Model file for the job. Use its own axes, mm. A direction names the side the tool comes from. Round coordinates to 2 decimals unless told otherwise and drop trailing zeros. Loops run counter-clockwise (first coordinate to the right, second up) from the corner with the lowest first, then second, coordinate; pieces in that order, holes last. Notation, with made-up numbers: (-27.75, 58) - (17.25, 58) arc R8 ccw to (17.25, 64) - close; hole circle Ø8 at (-17.75, -15). An arc over 180 degrees is marked (long way). Answer as a JSON object with one key per item and string values.
Autodesk Inventor part; units mm, degrees
ref_plane "YZ Plane" through (0, 0, 0) normal (1, 0, 0) x (0, 1, 0)
ref_plane "XZ Plane" through (0, 0, 0) normal (0, 1, 0) x (-1, 0, 0)
ref_plane "XY Plane" through (0, 0, 0) normal (0, 0, 1) x (1, 0, 0)
sketch "Sketch1" plane through (0, 0, 0) normal (0, 0, 1) x (1, 0, 0)
  line L0 (2.5344, 6.8804) -> (7.2258, 1.2453)
  line L1 (7.2258, 1.2453) -> (4.6914, -5.6351)
  line L2 (4.6914, -5.6351) -> (-2.5344, -6.8804)
  line L3 (-2.5344, -6.8804) -> (-7.2258, -1.2453)
  line L4 (-7.2258, -1.2453) -> (-4.6914, 5.6351)
  line L5 (-4.6914, 5.6351) -> (2.5344, 6.8804)
  line L6 (-1.847, 2.2185) -> (0.9978, 2.7088)
  line L7 (0.9978, 2.7088) -> (2.8448, 0.4903)
  line L8 (2.8448, 0.4903) -> (1.847, -2.2185)
  line L9 (1.847, -2.2185) -> (-0.9978, -2.7088)
  line L10 (-0.9978, -2.7088) -> (-2.8448, -0.4903)
  line L11 (-2.8448, -0.4903) -> (-1.847, 2.2185)
  point P0 (0, 0)
  point P1 (0, 0)
  point P2 (0, 0)
  dimension "d0" = 12.7
  dimension "d1" = 5
extrude "Extrusion1" add sketch "Sketch1" along normal blind 127
properties part number "cross beam"
1) Probe probe 1 along Y at (x, z) = (-1, 69); probe 2 along X at (y, z) = (-2, 121); probe 3 along Y at (x, z) = (1.5, 24.5). List the from-to ranges inside material, lowest first.
Values follow:
{"probe 1": "-6.62 to -2.71, 2.36 to 6.27", "probe 2": "-6.6 to -1.59, 1.93 to 6.03", "probe 3": "-6.19 to -2.28, 2.11 to 6.7"}
2) Tool access for faces 1 (the flat face through (5.976, -2.147, 62.611)), 2 (the flat face through (2.35, -0.85, 62.61)): list every direction of +Z, -Z, +X, -X, +Y, -Y with a clear straight run to the whole face (end or side of a thin tool).
Values follow:
{"face 1": "+Z, -Z, +X, -Y", "face 2": "+Z, -Z"}
3) Drop flat-ended pins along their axis: P1, Ø8, axis at y = -1, z = 65, coming from the -X side; P2, Ø4, axis at x = 0, z = 110.5, coming from the -Y side; P3, Ø4, axis at y = -5, z = 98.5, coming from the -X side. Give the stop position or say it passes through.
Values follow:
{"P1": "x = -7.23", "P2": "y = -6.79", "P3": "x = -5.76"}
4) Slice it at B-B on y = -4. List the corners of the cut face in (x, z).
Values follow:
{"outline": "(-4.93, 0) - (5.29, 0) - (5.29, 127) - (-4.93, 127) - close"}
5) Two-plate mould, pull along X, no slides. Class faces 3 (the flat face through (0, -3, 0)), 4 (the flat face through (-0.44, 2.46, 62.61)), 5 (the flat face through (-1.13, 6.25, 62.61)): pulls with the +X half, pulls with the -X half, needs draft (parallel to the pull), parting line crosses it, or undercut.
Values follow:
{"face 3": "needs draft", "face 4": "undercut", "face 5": "pulls with the -X half"}
6) Slice it at A-A on z = 41. List the corners of the cut face in (x, y).
Values follow:
{"outline": "(-7.23, -1.25) - (-2.53, -6.88) - (4.69, -5.64) - (7.23, 1.25) - (2.53, 6.88) - (-4.69, 5.64) - close; hole (-2.84, -0.49) - (-1, -2.71) - (1.85, -2.22) - (2.84, 0.49) - (1, 2.71) - (-1.85, 2.22) - close"}
